Geometry check sheet. Reference: the model listing, model coordinates, mm. Round coordinates to 2 decimals unless told otherwise and drop trailing zeros. Loops run counter-clockwise (first coordinate to the right, second up) from the corner with the lowest first, then second, coordinate; pieces in that order, holes last. Notation, with made-up numbers: (-25, -29) - (-3, -29) arc R8 ccw to (-3, -18) - close; hole circle Ø3 at (0, 67.25). An arc over 180 degrees is marked (long way). Answer as CSV lines item,"result". Start each with the question number.
1) Draft check along Y on faces 1 (the cylindrical face through (-111.1, -85.19, 1.97)), 2 (the cylindrical face through (30.374, 47.641, 2.465)), 3 (the flat face through (-2, -60, 0)). Enter one of: released by +Y, released by -Y, zero draft, split by the parting line, or undercut.
2) Thickness scan on line 1 along Y through (x, z) = (0, 3.7); line 2 along X through (y, z) = (8.5, 4.6); line 3 along X through (y, z) = (-38, 4.2). Record the ranges inside material, lowest first.
3) Depth check by flat-ended pin: P1, Ø1, axis at y = 102, z = 1.5, coming from the -X side; P2, Ø6, axis at x = 0, y = 130, coming from the +Z side; P3, Ø3, axis at x = -58.5, z = 4, coming from the -Y side; P4, Ø3, axis at y = 44, z = 1.5, coming from the -X side. Enter the tip coordinate at first touch or a pass-through.
4) Cross-section at A-A on z = 2.25. Record the boundary of the cut face in (x, y).
from build123d import *

# Parameters (mm, degrees)
SKETCH1_R                       = 140
SKETCH1_R_2                     = 56.5
BOSS_EXTRUDE1_DEPTH             = 5
F_5_0MM_DOWEL_HOLE1_D           = 5
F_5_0MM_DOWEL_HOLE1_CSINK_D     = 5.05
F_5_0MM_DOWEL_HOLE1_CSINK_ANGLE = 90
FILLET1_R                       = 1
CHAMFER1_SIZE                   = 1


with BuildPart() as part:
    # Sketch1 → Boss-Extrude1 (new body)
    with BuildSketch(Plane.XY):
        Circle(SKETCH1_R)
        Circle(SKETCH1_R_2, mode=Mode.SUBTRACT)
    extrude(amount=BOSS_EXTRUDE1_DEPTH)

    # Ø5.0mm Dowel Hole1 (through all)
    with Locations(Plane.XY.offset(5)):
        with Locations((0, 130), (0, -130), (130, 0), (-130, 0)):
            CounterSinkHole(F_5_0MM_DOWEL_HOLE1_D / 2, F_5_0MM_DOWEL_HOLE1_CSINK_D / 2, counter_sink_angle=F_5_0MM_DOWEL_HOLE1_CSINK_ANGLE)

    # Fillet1
    fillet1_edges = [part.edges().sort_by_distance(p)[0] for p in [
        (-140, 0, 5),
    ]]
    fillet(fillet1_edges, radius=FILLET1_R)

    # Chamfer1
    chamfer1_edges = [part.edges().sort_by_distance(p)[0] for p in [
        (-127.5, 0, 0),
        (132.5, 0, 0),
        (2.5, -130, 0),
        (2.5, 130, 0),
    ]]
    chamfer(chamfer1_edges, length=CHAMFER1_SIZE)


solid = part.part
Answer block:
1,face 1,"split by the parting line"
1,face 2,"undercut"
1,face 3,"zero draft"
2,line 1,"y = -140 to -132.5, -127.5 to -56.5, 56.5 to 127.5, 132.5 to 140"
2,line 2,"x = -139.54 to -55.86, 55.86 to 139.54"
2,line 3,"x = -134.72 to -41.81, 41.81 to 134.72"
3,P1,"stops at x = -96.42"
3,P2,"stops at z = 5"
3,P3,"stops at y = -127.87"
3,P4,"stops at x = -133.39"
4,outline,"circle Ø280 at (0, 0); hole circle Ø5 at (-130, 0); hole circle Ø113 at (0, 0); hole circle Ø5 at (0, -130); hole circle Ø5 at (0, 130); hole circle Ø5 at (130, 0)"
